```python
from build123d import *

# Parameters (mm, degrees)
F1_DEPTH       = 12.7
F3_D           = 5.5
F3_CBORE_D     = 9.75
F3_CBORE_DEPTH = 5
F4_R           = 6.336218
F5_DEPTH       = 25.4
F8_DEPTH       = 1.5875


with BuildPart() as f1:
    # F0 (on Top) → F1 (new body)
    with BuildSketch(Plane.XY):
        Polygon((-0.584762, -44.992867), (38.672585, -23.002853), (39.257347, 21.990015), (0.584762, 44.992867), (-38.672585, 23.002853), (-39.257347, -21.990015), align=None)
    extrude(amount=-F1_DEPTH)

    # F3 (through all)
    with Locations(Plane.XY):
        with Locations((0, -36.943253), (31.830151, 0), (0, 36.042843), (-32.459036, 0)):
            CounterBoreHole(F3_D / 2, F3_CBORE_D / 2, F3_CBORE_DEPTH)

    # F4 (on Top) → F5 (cut)
    with BuildSketch(Plane.XY):
        Circle(F4_R)
    extrude(amount=-F5_DEPTH, mode=Mode.SUBTRACT)

    # F7 (on offset) → F8 (cut)
    with BuildSketch(Plane.XY.offset(-12.7)):
        Polygon((36.793541, 20.338582), (0.783042, 42.033432), (-36.010499, 21.69485), (-36.793541, -20.338582), (-0.783042, -42.033432), (36.010499, -21.69485), align=None)
    extrude(amount=F8_DEPTH, mode=Mode.SUBTRACT)


solid = f1.part
```
The listing builds one solid part. Answer for the finished solid, in the listing's coordinates (mm). A direction names the side the tool comes from. Give positions to 0.01 mm unless a question says otherwise; leave off trailing zeros. Order: outer loops, then holes, each group sorted by start corner. A loop starts at its lowest first (then second) coordinate and runs counter-clockwise, first axis right, second up. Notation, with made-up numbers: (-15, 73.5) - (35, 73.5) arc R30 cw to (35, 97.5) - close; hole circle Ø8 at (64, 82). An arc over 180 degrees is marked (long way). Use one line per item in the form item = value. Start each with the question number.
(1) Flat-ended cylindrical pins translate along their axes: pin 1 Ø5 at (x, y) = (3.5, 26) entering from -Z; pin 2 Ø11 at (x, y) = (31.83, 0) entering from -Z; pin 3 Ø5 at (y, z) = (3, -7.5) entering from +X; pin 4 Ø9 at (x, y) = (0, -36.94) entering from +Z. Find the tip coordinate at first contact, or state that the pin passes through.
(2) The mould has two halves that part along Y. Classify faces 4 (the flat face through (18.77, -34.15, -6.26)), 5 (the flat face through (2.1, -39, -5)), 6 (the flat face through (-18.77, 34.15, -6.26)): released by +Y, released by -Y, zero draft, split by the parting line, or undercut.
(3) A cutting plane is placed at C-C, the plane z = -4. Write down the section's boundary in (x, y) (3 decimals).
(4) Consider line 1 (Y direction, x = 0, z = -3.35); line 2 (Y direction, x = 0, z = -9); line 3 (Z direction, x = 4, y = -39.5). Determine where each line is inside the solid, lowest interval first. Write a range as from..to.
(5) A cutting plane is placed at A-A, the plane y = 0. Write down the section's boundary in (x, z).
(6) A cutting plane is placed at B-B, the plane x = -32. Write down the section's boundary in (y, z).
(7) For faces 1 (the flat face through (-20.19, -33.33, -6.26)), 2 (the flat face through (-1, -9, -11.112)), 3 (the cylindrical face through (36.48, 1.46, -2.46)), determine the directions among +Z, -Z, +X, -X, +Y, -Y from which every point of the face is accessible in a straight line to the end or side of a thin tool.
(8) A cutting plane is placed at D-D, the plane x = 23. Write down the section's boundary in (y, z).
Ans:
q1.pin_1 = -11.11
q1.pin_2 = -12.7
q1.pin_3 = 39.04
q1.pin_4 = -5
q2.face_4 = released by -Y
q2.face_5 = undercut
q2.face_6 = released by +Y
q3.outline = (-39.257, -21.99) - (-0.585, -44.993) - (38.673, -23.003) - (39.257, 21.99) - (0.585, 44.993) - (-38.673, 23.003) - close; hole circle Ø9.75 at (-32.459, 0); hole circle Ø12.672 at (0, 0); hole circle Ø9.75 at (0, -36.943); hole circle Ø9.75 at (0, 36.043); hole circle Ø9.75 at (31.83, 0)
q4.line_1 = -44.67..-41.82, -32.07..-6.34, 6.34..31.17, 40.92..44.67
q4.line_2 = -44.67..-39.69, -34.19..-6.34, 6.34..33.29, 38.79..44.67
q4.line_3 = -12.7..-5
q5.outline = (-38.97, -12.7) - (-36.41, -12.7) - (-36.41, -11.11) - (-35.21, -11.11) - (-35.21, -5) - (-37.33, -5) - (-37.33, 0) - (-38.97, 0) - close; (-29.71, -11.11) - (-6.34, -11.11) - (-6.34, 0) - (-27.58, 0) - (-27.58, -5) - (-29.71, -5) - close; (6.34, -11.11) - (29.08, -11.11) - (29.08, -5) - (26.96, -5) - (26.96, 0) - (6.34, 0) - close; (34.58, -11.11) - (36.41, -11.11) - (36.41, -12.7) - (38.97, -12.7) - (38.97, 0) - (36.71, 0) - (36.71, -5) - (34.58, -5) - close
q6.outline = (-26.31, -12.7) - (-23.23, -12.7) - (-23.23, -11.11) - (-2.71, -11.11) - (-2.71, -5) - (-4.85, -5) - (-4.85, 0) - (-26.31, 0) - close; (2.71, -11.11) - (23.91, -11.11) - (23.91, -12.7) - (26.74, -12.7) - (26.74, 0) - (4.85, 0) - (4.85, -5) - (2.71, -5) - close
q7.face_1 = +Z, -Z, -X, -Y
q7.face_2 = -Z
q7.face_3 = +Z
q8.outline = (-31.78, -12.7) - (-28.89, -12.7) - (-28.89, -11.11) - (28.65, -11.11) - (28.65, -12.7) - (31.66, -12.7) - (31.66, 0) - (-31.78, 0) - close
